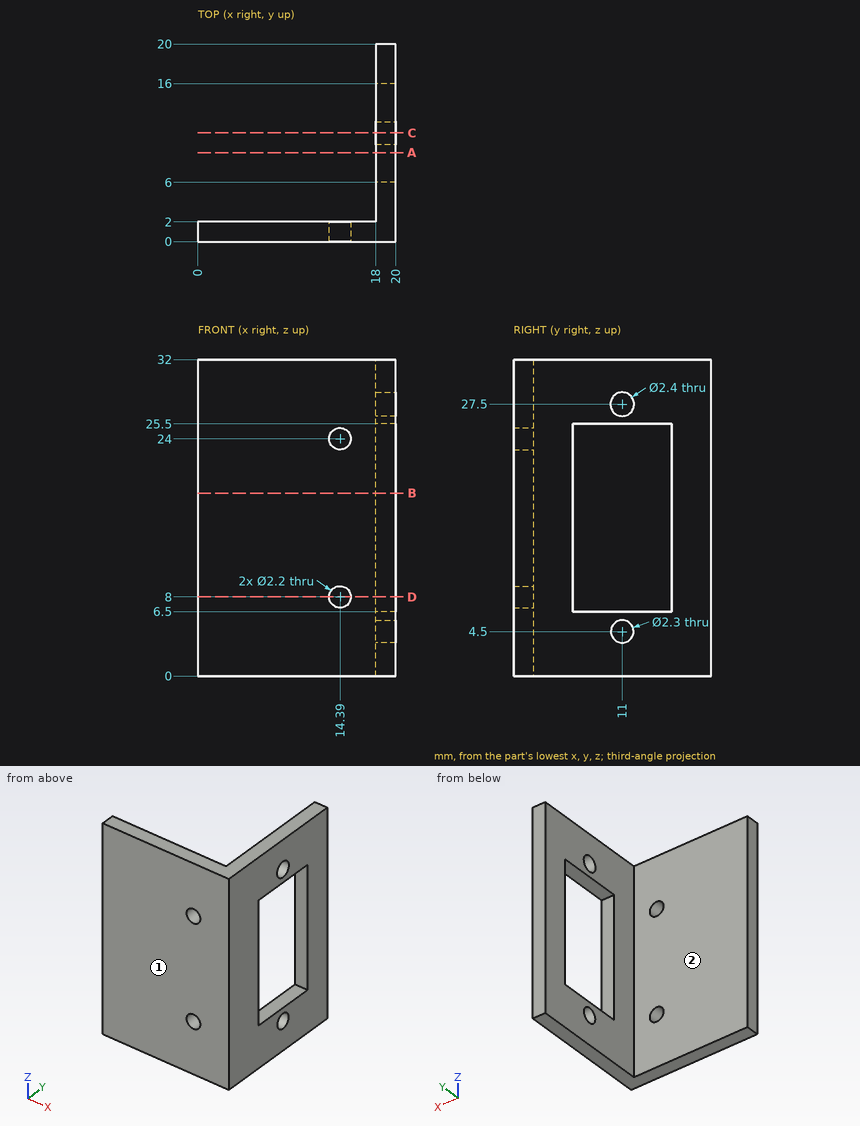
Can you work these out from the drawing? Everything is in mm from the part's minimum corner. A direction names the side the tool comes from. Coordinates: 2 decimals unless noted, no trailing zeros. Write each loop counter-clockwise with the first axis right and the second up, starting at its lowest first coordinate (ties: lowest second). Pieces come first, ordered by that corner, then holes. Notation, with made-up numbers: (-15.5, 39.25) -> (29.5, 39.25) arc R28 ccw to (29.5, 78.25) -> close; hole circle Ø3 at (2, 62). An arc over 180 degrees is marked (long way). Write each question's results on one line, items separated by ' | '. Start each with the question number.
Q1. Imagine slicing it at C-C (y = 11). Write out the boundary of the cut face in (x, z), then the cut area to 3 significant figures.
Q2. Imagine slicing it at B-B (z = 18.5). Write out the boundary of the cut face in (x, y).
Q3. I'm going to push flat-ended pins straight in: pin 1 (3 mm diameter, centred on y = 14, z = 23, fed in from -X); pin 2 (1 mm diameter, centred on y = 17.5, z = 18.5, fed in from -X). Where does each tip first touch, or does it pass through?
Q4. On a 3-axis mill with a long thin cutter (end or side, diameter ignored), from which of +Z, -Z, +X, -X, +Y, -Y can I reach the whole of each face in a straight line? I mean the marked faces 1 and 2. Say none if no direction works.
Q5. Imagine slicing it at A-A (y = 9). Write out the boundary of the cut face in (x, z).
Q6. Imagine slicing it at D-D (z = 8). Write out the boundary of the cut face in (x, y), then the cut area to 3 significant figures.
Q7. If I drill on probe 1 along Y at (x, z) = (18.5, 27.5); probe 2 along X at (y, z) = (1.45, 8); probe 3 along Y at (x, z) = (18.25, 13.5), over which ranges is the centre line in solid material (lowest first)?
Taken from the geometry:
1) outline: (18, 0) -> (20, 0) -> (20, 3.35) -> (18, 3.35) -> close; (18, 5.65) -> (20, 5.65) -> (20, 6.5) -> (18, 6.5) -> close; (18, 25.5) -> (20, 25.5) -> (20, 26.3) -> (18, 26.3) -> close; (18, 28.7) -> (20, 28.7) -> (20, 32) -> (18, 32) -> close | area: 16.6 mm^2
2) outline: (0, 0) -> (20, 0) -> (20, 6) -> (18, 6) -> (18, 2) -> (0, 2) -> close; (18, 16) -> (20, 16) -> (20, 20) -> (18, 20) -> close
3) pin 1: passes through | pin 2: stops at x = 18
4) face 1: +Z, -Z, +X, -X, -Y | face 2: +Z, -Z, -X, +Y
5) outline: (18, 0) -> (20, 0) -> (20, 6.5) -> (18, 6.5) -> close; (18, 25.5) -> (20, 25.5) -> (20, 32) -> (18, 32) -> close
6) outline: (0, 0) -> (13.29, 0) -> (13.29, 2) -> (0, 2) -> close; (15.49, 0) -> (20, 0) -> (20, 6) -> (18, 6) -> (18, 2) -> (15.49, 2) -> close; (18, 16) -> (20, 16) -> (20, 20) -> (18, 20) -> close | area: 51.6 mm^2
7) probe 1: y = 0 to 9.8, 12.2 to 20 | probe 2: x = 0 to 13.29, 15.49 to 20 | probe 3: y = 0 to 6, 16 to 20
